```python
from build123d import *

# Parameters (mm, degrees)
SKETCH1_W           = 30
SKETCH1_H           = 8
SKETCH1_R           = 1.725
BOSS_EXTRUDE1_DEPTH = 4
FILLET1_R           = 3


with BuildPart() as part:
    # Sketch1 → Boss-Extrude1 (new body)
    with BuildSketch(Plane(origin=(0, 0, 0), x_dir=(1, 0, 0), z_dir=(0, 1, 0))):
        with Locations((10, 0)):
            Rectangle(SKETCH1_W, SKETCH1_H)
        with Locations(Location((0, 0, 0), (0, 0, 270))):
            Circle(SKETCH1_R, mode=Mode.SUBTRACT)
        with Locations(Location((20, 0, 0), (0, 0, 270))):
            Circle(SKETCH1_R, mode=Mode.SUBTRACT)
    extrude(amount=BOSS_EXTRUDE1_DEPTH)

    # Fillet1
    fillet1_edges = [part.edges().sort_by_distance(p)[0] for p in [
        (25, 2, 4),
        (-5, 2, 4),
    ]]
    fillet(fillet1_edges, radius=FILLET1_R)


solid = part.part
```
Here's how the part is built. I have some questions about the finished solid (model axes, mm). Coordinates: 2 decimals unless noted, no trailing zeros. Write each loop counter-clockwise with the first axis right and the second up, starting at its lowest first coordinate (ties: lowest second). Pieces come first, ordered by that corner, then holes. Notation, with made-up numbers: M 64.5,48 L 101.5,48 A20 ccw 101.5,62 Z; hole C 68.5,67.5 d3. An arc over 180 degrees is marked long. Answer as CSV lines item,"result". Start each with the question number.
Q1. I need wall thicknesses on probe 1 along X at (y, z) = (3.15, 0) (3 decimals); probe 2 along Z at (x, y) = (-0.5, 0.95); probe 3 along Z at (x, y) = (0.75, 1.7). Which ranges of each line are inside material? Lowest first, please. Write a range as [from, to].
Q2. Suppose I cut it at A-A, the plane x = 0. List the corners of the cut face in (y, z) for me (3 decimals).
Q3. Will this pin go through, and if not, where does the flat tip stop? pin 1 Ø1 at (y, z) = (1.5, 3) entering from -X.
Q4. Suppose I cut it at B-B, the plane z = 0. List the corners of the cut face in (x, y) for me (3 decimals).
Q5. Suppose I cut it at C-C, the plane y = 2.5. List the corners of the cut face in (x, z) for me (3 decimals).
Q6. If we mould it in two halves opening along Z, with no side actions, what happens to faces 1 (the cylindrical face through (18.316, 1.972, -0.374)), 2 (the flat face through (25, 2, -1)), 3 (the cylindrical face through (24.1, 2.03, 3.14)), 4 (the flat face through (10, 2, -4))? For each: pulls with the +Z half, pulls with the -Z half, needs draft (parallel to the pull), parting line crosses it, or undercut.
Entries:
1,probe 1,"x = [-5, -1.725], [1.725, 18.275], [21.725, 25]"
1,probe 2,"z = [-4, -1.65], [1.65, 4]"
1,probe 3,"z = [-4, -1.55], [1.55, 4]"
2,outline,"M 0,-4 L 4,-4 L 4,-1.725 L 0,-1.725 Z; M 0,1.725 L 4,1.725 L 4,4 L 0,4 Z"
3,pin 1,"stops at x = -4.6"
4,outline,"M -5,0 L -1.725,0 L -1.725,4 L -5,4 Z; M 1.725,0 L 18.275,0 L 18.275,4 L 1.725,4 Z; M 21.725,0 L 25,0 L 25,4 L 21.725,4 Z"
5,outline,"M -5,-4 L 25,-4 L 25,1 A3 ccw 22,4 L -2,4 A3 ccw -5,1 Z; hole C 0,0 d3.45; hole C 20,0 d3.45"
6,face 1,"undercut"
6,face 2,"needs draft"
6,face 3,"pulls with the +Z half"
6,face 4,"pulls with the -Z half"
